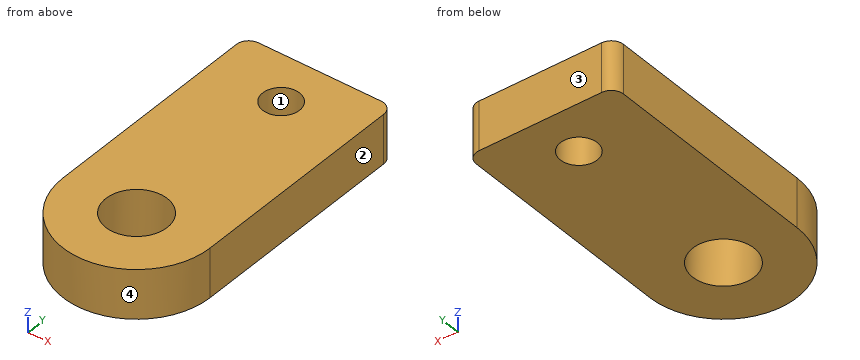
from build123d import *

# Parameters (mm, degrees)
SKETCH_R   = 2.5
SKETCH_R_2 = 1.5
PAD_DEPTH  = 4
FILLET_R   = 1


with BuildPart() as part:
    # Sketch → Pad (new body)
    with BuildSketch(Plane.XY):
        with BuildLine():
            ThreePointArc((-6, 0), (0, -6), (6, 0))
            Line((6, 0), (6, 19))
            Line((6, 19), (-6, 19))
            Line((-6, 0), (-6, 19))
        make_face()
        Circle(SKETCH_R, mode=Mode.SUBTRACT)
        with Locations((0, 15)):
            Circle(SKETCH_R_2, mode=Mode.SUBTRACT)
    extrude(amount=PAD_DEPTH)

    # Fillet
    fillet_edges = [part.edges().sort_by_distance(p)[0] for p in [
        (-6, 19, 2),
        (6, 19, 2),
    ]]
    fillet(fillet_edges, radius=FILLET_R)


solid = part.part
Verification items for the finished model (mm, model axes). Face numbers are marked on the shaded views. Coordinates: 2 decimals unless noted, no trailing zeros. Order: outer loops, then holes, each group sorted by start corner. A loop starts at its lowest first (then second) coordinate and runs counter-clockwise, first axis right, second up.
Item 1: Material ranges on L1, parallel to Y at x = 0, z = 1.3; L2, parallel to Y at x = -1, z = 0.85; L3, parallel to Y at x = -2, z = 1.85, recorded low to high.
Filled in:
L1: y = -6 to -2.5, 2.5 to 13.5, 16.5 to 19
L2: y = -5.92 to -2.29, 2.29 to 13.88, 16.12 to 19
L3: y = -5.66 to -1.5, 1.5 to 19
Item 2: Section check D-D, the plane y = -1. Enter the section's corners in (x, z), then the cut area to 3 significant figures.
Filled in:
outline: (-5.92, 0) - (-2.29, 0) - (-2.29, 4) - (-5.92, 4) - close; (2.29, 0) - (5.92, 0) - (5.92, 4) - (2.29, 4) - close
area: 29.0 mm2
Item 3: Section check C-C, the plane z = 2.9. Enter the section's corners in (x, y).
Filled in:
outline: (-6, 0) arc R6 ccw to (6, 0) - (6, 18) arc R1 ccw to (5, 19) - (-5, 19) arc R1 ccw to (-6, 18) - close; hole circle Ø5 at (0, 0); hole circle Ø3 at (0, 15)
Item 4: Section check A-A, the plane y = 15. Enter the section's corners in (x, z).
Filled in:
outline: (-6, 0) - (-1.5, 0) - (-1.5, 4) - (-6, 4) - close; (1.5, 0) - (6, 0) - (6, 4) - (1.5, 4) - close
Item 5: Depth check by flat-ended pin: pin 1 (1.8 mm diameter, centred on x = 0, y = 15, fed in from +Z). Enter the tip coordinate at first touch or a pass-through.
Filled in:
pin 1: passes through
Item 6: Section check B-B, the plane x = 0. Enter the section's corners in (y, z).
Filled in:
outline: (-6, 0) - (-2.5, 0) - (-2.5, 4) - (-6, 4) - close; (2.5, 0) - (13.5, 0) - (13.5, 4) - (2.5, 4) - close; (16.5, 0) - (19, 0) - (19, 4) - (16.5, 4) - close
Item 7: Release check for a two-part mould opening along X. For the marked faces 1, 2, 3 and 4 record: +X half, -X half, draft (parallel to the pull), parting line (faces both ways), or undercut.
Filled in:
face 1: undercut
face 2: +X half
face 3: draft
face 4: parting line
